Can you work these out from the model? Positions are in its coordinate system, mm. Round coordinates to 2 decimals unless told otherwise and drop trailing zeros. Loops run counter-clockwise (first coordinate to the right, second up) from the corner with the lowest first, then second, coordinate; pieces in that order, holes last. Notation, with made-up numbers: M 13.25,20 L 72.25,20 A31 cw 72.25,44 Z; hole C -16.5,27.25 d2. An arc over 180 degrees is marked long. Use a Markdown table: item, result. Add a question column.
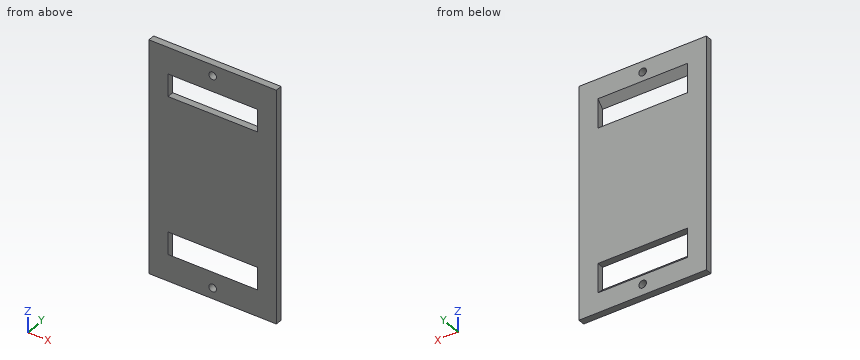
```python
from build123d import *

# Parameters (mm, degrees)
SKETCH_1_W          = 57
SKETCH_1_H          = 103.6
SKETCH_1_R          = 1.7
EXTRUDE_1_DEPTH     = 3
SKETCH_2_W          = 40
SKETCH_2_H          = 10
CUT_EXTRUDE_1_DEPTH = 3
CHAMFER_1_SIZE      = 3


with BuildPart() as part:
    # 草图1 → 凸台-拉伸1 (new body)
    with BuildSketch(Plane(origin=(0, 0, 0), x_dir=(1, 0, 0), z_dir=(0, 1, 0))):
        Rectangle(SKETCH_1_W, SKETCH_1_H)
        with Locations(Location((0, 47, 0), (0, 0, 270))):
            Circle(SKETCH_1_R, mode=Mode.SUBTRACT)
        with Locations(Location((0, -47, 0), (0, 0, 270))):
            Circle(SKETCH_1_R, mode=Mode.SUBTRACT)
    extrude(amount=EXTRUDE_1_DEPTH)

    # 草图2 → 切除-拉伸1 (cut)
    with BuildSketch(Plane(origin=(0, 3, 0), x_dir=(1, 0, 0), z_dir=(0, 1, 0))):
        with Locations((0, 35)):
            Rectangle(SKETCH_2_W, SKETCH_2_H)
        with Locations((0, -35)):
            Rectangle(SKETCH_2_W, SKETCH_2_H)
    extrude(amount=-CUT_EXTRUDE_1_DEPTH, mode=Mode.SUBTRACT)

    # 倒角1
    chamfer_1_edges = [part.edges().sort_by_distance(p)[0] for p in [
        (0, 3, 40),
        (0, 3, -40),
    ]]
    chamfer(chamfer_1_edges, length=CHAMFER_1_SIZE - 0.0001)  # a hair under: the kernel refuses the full size


solid = part.part
```
(1) Suppose I cut it at B-B on z = -47. List the corners of the cut face in (x, y) for me, and give its area (3 significant figures).
(2) Suppose I cut it at A-A on x = 0. Count the separate pieces of the cut face and the enclosed holes in it, and give its area (3 significant figures).
(3) I'm going to push a flat-ended pin straight in: pin 1 (3 mm diameter, centred on x = 0, z = 47, fed in from +Y). Where does the tip first touch, or does it pass through?
(4) Suppose I cut it at C-C on y = 1.85. List the corners of the cut face in (x, z) for me.
(5) If I drill on probe 1 along X at (y, z) = (0.3, 31); probe 2 along Z at (x, y) = (-17, 0.55); probe 3 along Z at (x, y) = (-16, 2.1), over which ranges is the centre line in solid material (lowest first)? Write a range as [from, to].
Results below:
| question | item | result |
|---|---|---|
| 1 | outline | M -28.5,0 L -1.7,0 L -1.7,3 L -28.5,3 Z; M 1.7,0 L 28.5,0 L 28.5,3 L 1.7,3 Z |
| 1 | area | 161 mm² |
| 2 | separate pieces | 5 |
| 2 | enclosed holes | 0 |
| 2 | area | 221 mm² |
| 3 | pin 1 | passes through |
| 4 | outline | M -28.5,-51.8 L 28.5,-51.8 L 28.5,51.8 L -28.5,51.8 Z; hole M -20,-41.85 L 20,-41.85 L 20,-30 L -20,-30 Z; hole M -20,30 L 20,30 L 20,41.85 L -20,41.85 Z; hole C 0,-47 d3.4; hole C 0,47 d3.4 |
| 5 | probe 1 | x = [-28.5, -20], [20, 28.5] |
| 5 | probe 2 | z = [-51.8, -40.55], [-30, 30], [40.55, 51.8] |
| 5 | probe 3 | z = [-51.8, -42.1], [-30, 30], [42.1, 51.8] |
